Geometry check sheet. Reference: drawing and pictorial views, mm from the part's lowest x, y, z. Coordinates: 2 decimals unless noted, no trailing zeros. Loops run counter-clockwise (first coordinate to the right, second up) from the corner with the lowest first, then second, coordinate; pieces in that order, holes last. Notation, with made-up numbers: (7.5, 81.5) -> (25.5, 81.5) arc R33 ccw to (25.5, 119.5) -> close; hole circle Ø4 at (3, 78). An arc over 180 degrees is marked (long way). Use one line per item in the form item = value.
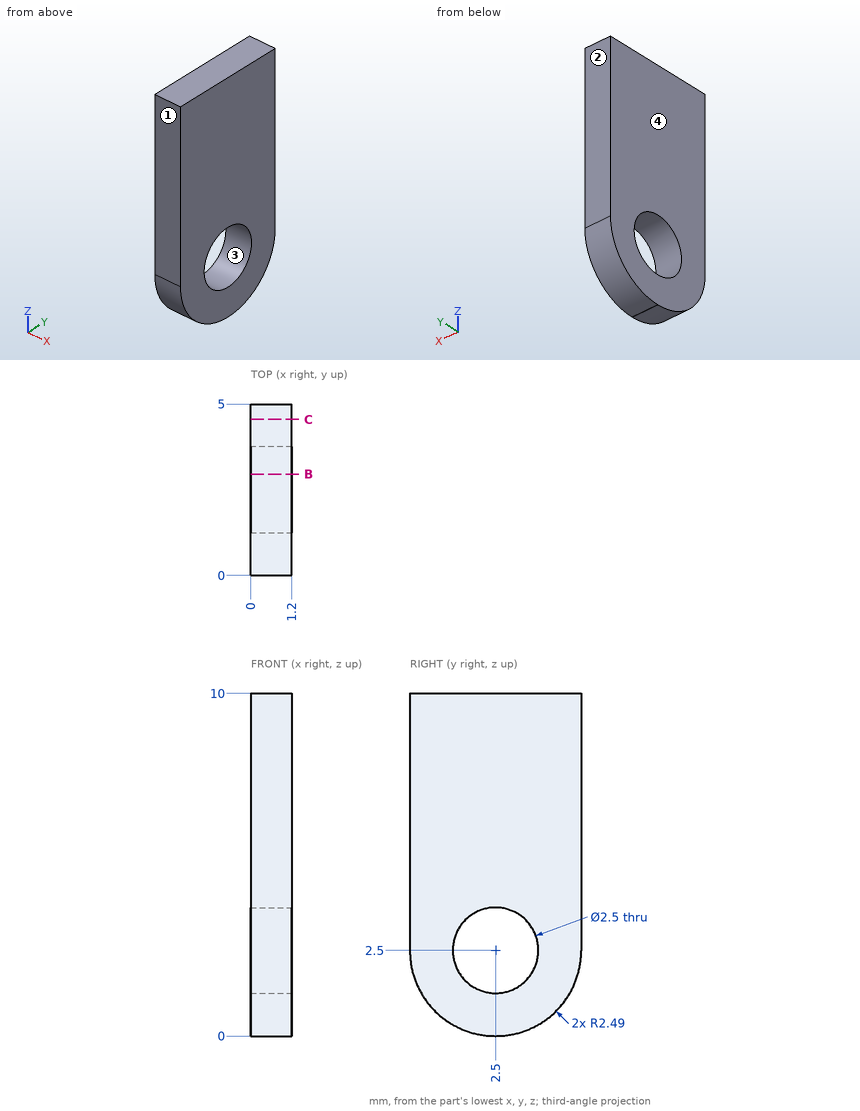
(1) Mould release check, pull along Y, two halves, no side actions. Record for the marked faces 1, 2, 3 and 4: +Y half, -Y half, draft (parallel to the pull), parting line (faces both ways), or undercut.
Established:
face_1 = -Y half
face_2 = +Y half
face_3 = undercut
face_4 = draft
(2) Scan lines: line 1 along Z through (x, y) = (0.95, 2.5); line 2 along Y through (x, z) = (0.35, 2.25); line 3 along Z through (x, y) = (0.6, 1.4). Record each from-to range of solid material in increasing order.
Established:
line_1 = 0 to 1.25, 3.75 to 10
line_2 = 0.01 to 1.28, 3.72 to 4.99
line_3 = 0.25 to 1.91, 3.09 to 10
(3) Section check B-B, the plane y = 2.95. Record the boundary of the cut face in (x, z), plus the area to 3 significant figures.
Established:
outline = (0, 0.04) -> (1.2, 0.04) -> (1.2, 1.33) -> (0, 1.33) -> close; (0, 3.67) -> (1.2, 3.67) -> (1.2, 10) -> (0, 10) -> close
area = 9.15 mm²
(4) Section check C-C, the plane y = 4.55. Record the boundary of the cut face in (x, z).
Established:
outline = (0, 1.06) -> (1.2, 1.06) -> (1.2, 10) -> (0, 10) -> close
